Read the model definition and answer for the solid it produces. Units are mm, in the model's axes. Face numbers are marked on the shaded views. A direction names the side the tool comes from. Coordinates: 2 decimals unless noted, no trailing zeros. Order: outer loops, then holes, each group sorted by start corner. A loop starts at its lowest first (then second) coordinate and runs counter-clockwise, first axis right, second up. Notation, with made-up numbers: M -10.5,-30.75 L 38.5,-30.75 A19 ccw 38.5,-26.75 Z; hole C 15.25,23 d3. An arc over 180 degrees is marked long. Use a Markdown table: item, result. Add a question column.
1) Find section A-A on x = -15. Write down the section's boundary in (y, z).
2) This flat-tipped pin is pushed along its axis until it touches: pin 1 Ø5 at (x, y) = (-49, 34.5) entering from +Z. Where does it stop, or does it pass through?
3) The mould has two halves that part along Y. Classify the marked faces 3, 4, 5 and 6: released by +Y, released by -Y, zero draft, split by the parting line, or undercut.
4) Find the intervals of material crossed by probe 1 along Y at (x, z) = (-45, 0.7); probe 2 along Y at (x, z) = (-51.5, 14.25); probe 3 along X at (y, z) = (16, 5.5), in increasing order. Write a range as [from, to].
5) Find section C-C on y = -15. Write down the section's boundary in (x, z).
6) Find section B-B on y = -2. Write down the section's boundary in (x, z).
7) For the marked faces 1 and 2, determine the directions among +Z, -Z, +X, -X, +Y, -Y from which every point of the face is accessible in a straight line to the end or side of a thin tool.
from build123d import *

# Parameters (mm, degrees)
F1_W     = 150
F1_H     = 66
F2_DEPTH = 20
F3_DEPTH = 3
F4_R     = 2.7
F6_DEPTH = 25
F5_W     = 10
F5_H     = 6.4
F7_DEPTH = 160
F8_R     = 5
F9_R     = 1
F10_SIZE = 0.5


with BuildPart() as f2:
    # F1 (on Top) → F2 (new body)
    with BuildSketch(Plane.XY):
        with Locations((0, 10)):
            Rectangle(F1_W, F1_H)
        with BuildLine():
            Line((70, 23.1270166538), (70, 20.0717967697))
            Line((70, 20.0717967697), (70, -13))
            Line((70, -13), (70, -18))
            Line((70, -18), (65, -18))
            Line((65, -18), (-65, -18))
            Line((-65, -18), (-70, -18))
            Line((-70, -18), (-70, -13))
            Line((-70, -13), (-70, 30))
            Line((-70, 30), (-70, 38))
            Line((-70, 38), (-48.8729833462, 38))
            ThreePointArc((-48.8729833462, 38), (-45, 41), (-41.1270166538, 38))
            Line((-41.1270166538, 38), (-38.0717967697, 38))
            Line((-38.0717967697, 38), (62, 38))
            Line((62, 38), (70, 38))
            Line((70, 38), (70, 30.8729833462))
            ThreePointArc((70, 30.8729833462), (72.1622776602, 29.4494897428), (73, 27))
            ThreePointArc((73, 27), (72.1622776602, 24.5505102572), (70, 23.1270166538))
        make_face(mode=Mode.SUBTRACT)
    extrude(amount=F2_DEPTH)

    # F1 (on Top) → F3 (join)
    with BuildSketch(Plane.XY):
        with BuildLine():
            ThreePointArc((-45, 30), (-39.7084973779, 32.417424305), (-38.0717967697, 38))
            Line((-38.0717967697, 38), (-41.1270166538, 38))
            ThreePointArc((-41.1270166538, 38), (-41.0318812149, 37.5040171699), (-41, 37))
            ThreePointArc((-41, 37), (-45.5040171699, 33.0318812149), (-48.8729833462, 38))
            Line((-48.8729833462, 38), (-70, 38))
            Line((-70, 38), (-70, 30))
            Line((-70, 30), (-45, 30))
        make_face()
        with BuildLine():
            ThreePointArc((62, 27), (64.417424305, 21.7084973779), (70, 20.0717967697))
            Line((70, 20.0717967697), (70, 23.1270166538))
            ThreePointArc((70, 23.1270166538), (65, 27), (70, 30.8729833462))
            Line((70, 30.8729833462), (70, 38))
            Line((70, 38), (62, 38))
            Line((62, 38), (62, 27))
        make_face()
        with BuildLine():
            Line((70, 25.2679491924), (70, 23.1270166538))
            ThreePointArc((70, 23.1270166538), (72.1622776602, 24.5505102572), (73, 27))
            ThreePointArc((73, 27), (72.1622776602, 29.4494897428), (70, 30.8729833462))
            Line((70, 30.8729833462), (70, 28.7320508076))
            ThreePointArc((70, 28.7320508076), (70.7320508076, 28), (71, 27))
            ThreePointArc((71, 27), (70.7320508076, 26), (70, 25.2679491924))
        make_face()
        with BuildLine():
            ThreePointArc((70, 30.8729833462), (65, 27), (70, 23.1270166538))
            Line((70, 23.1270166538), (70, 25.2679491924))
            ThreePointArc((70, 25.2679491924), (67, 27), (70, 28.7320508076))
            Line((70, 28.7320508076), (70, 30.8729833462))
        make_face()
        with BuildLine():
            ThreePointArc((-41, 37), (-41.0318812149, 37.5040171699), (-41.1270166538, 38))
            Line((-41.1270166538, 38), (-43.2679491924, 38))
            ThreePointArc((-43.2679491924, 38), (-43.0681483474, 37.5176380902), (-43, 37))
            ThreePointArc((-43, 37), (-45.5176380902, 35.0681483474), (-46.7320508076, 38))
            Line((-46.7320508076, 38), (-48.8729833462, 38))
            ThreePointArc((-48.8729833462, 38), (-45.5040171699, 33.0318812149), (-41, 37))
        make_face()
        with BuildLine():
            Line((-43.2679491924, 38), (-41.1270166538, 38))
            ThreePointArc((-41.1270166538, 38), (-45, 41), (-48.8729833462, 38))
            Line((-48.8729833462, 38), (-46.7320508076, 38))
            ThreePointArc((-46.7320508076, 38), (-45, 39), (-43.2679491924, 38))
        make_face()
        Polygon((-70, -18), (-65, -18), (-70, -13), align=None)
        Polygon((70, -18), (70, -13), (65, -18), align=None)
    extrude(amount=F3_DEPTH)

    # F4 (on face) → F6 (cut)
    with BuildSketch(Plane.XZ.offset(23)):
        with Locations((-50, 10)):
            Circle(F4_R)
        with Locations((50, 10)):
            Circle(F4_R)
    extrude(amount=-F6_DEPTH, mode=Mode.SUBTRACT)

    # F5 (on face) → F7 (cut)
    with BuildSketch(Plane(origin=(-75, 0, 0), x_dir=(0, -1, 0), z_dir=(-1, 0, 0))):
        with Locations((-15, 10)):
            Rectangle(F5_W, F5_H)
    extrude(amount=-F7_DEPTH, mode=Mode.SUBTRACT)

    # F8
    f8_edges = [f2.edges().sort_by_distance(p)[0] for p in [
        (62, 38, 1.5),
        (-70, 30, 1.5),
        (70, 38, 11.5),
        (-70, 38, 11.5),
        (-70, -18, 11.5),
        (70, -18, 11.5),
        (-38.071797, 38, 1.5),
        (70, 20.071797, 1.5),
    ]]
    fillet(f8_edges, radius=F8_R)

    # F9
    f9_edges = [f2.edges().sort_by_distance(p)[0] for p in [
        (-75, 43, 10),
        (-75, -23, 10),
        (75, -23, 10),
        (75, 43, 10),
        (-72.5, 10, 6.8),
        (-72.5, 20, 6.8),
        (72.5, 20, 6.8),
        (72.5, 10, 6.8),
    ]]
    fillet(f9_edges, radius=F9_R)

    # F10
    f10_edges = [f2.edges().sort_by_distance(p)[0] for p in [
        (-72.5, 10, 13.2),
        (-72.5, 20, 13.2),
        (72.5, 20, 13.2),
        (72.5, 10, 13.2),
    ]]
    chamfer(f10_edges, length=F10_SIZE)


solid = f2.part
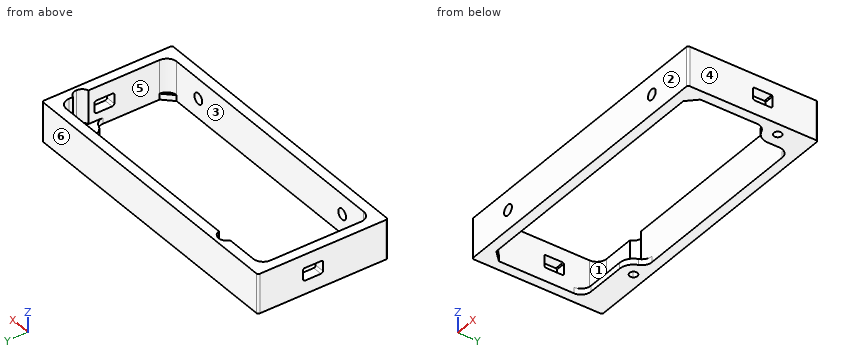
Check result:
| question | item | result |
|---|---|---|
| 1 | outline | M -23,0 L -18,0 L -18,20 L -23,20 Z; M 38,0 L 43,0 L 43,20 L 38,20 Z |
| 2 | pin 1 | stops at z = 3 |
| 3 | face 3 | undercut |
| 3 | face 4 | zero draft |
| 3 | face 5 | undercut |
| 3 | face 6 | released by +Y |
| 4 | probe 1 | y = [-23, -18], [30, 35], [39, 43] |
| 4 | probe 2 | y = [-23, -18], [38, 43] |
| 4 | probe 3 | x = [-75, -70], [70, 75] |
| 5 | outline | M -75,0 L -68,0 L -68,3 L -69.58,3 L -69.58,20 L -75,20 Z; M 68,0 L 75,0 L 75,20 L 69.58,20 L 69.58,3 L 68,3 Z |
| 6 | outline | M -75,0 L -70,0 L -70,20 L -75,20 Z; M 70,0 L 75,0 L 75,20 L 70,20 Z |
| 7 | face 1 | +Z |
| 7 | face 2 | +Z, -Z, +X, -X, -Y |
